from build123d import *

# Parameters (mm, degrees)
RESSALTO_EXTRUS_O1_DEPTH                             = 4
FILETE1_R                                            = 4
CHANFRO1_SIZE                                        = 1
FURO_DE_DI_METRO_6_0_6_1_D                           = 6
ESCAREADO_PARA_PARAFUSO_COM_CABE_A_ESCAR_D           = 3.4
ESCAREADO_PARA_PARAFUSO_COM_CABE_A_ESCAR_CSINK_D     = 6.3
ESCAREADO_PARA_PARAFUSO_COM_CABE_A_ESCAR_CSINK_ANGLE = 90
BROCA_DE_ROSQUEAR_PARA_TARRAXA_DE_M21_D              = 1.6
BROCA_DE_ROSQUEAR_PARA_TARRAXA_DE_M21_DEPTH          = 10
BROCA_DE_ROSQUEAR_PARA_TARRAXA_DE_M21_TIP            = 0.480688495
ESCAREADO_PARA_PARAFUSO_COM_CABE_A_E_2_D             = 3.4
ESCAREADO_PARA_PARAFUSO_COM_CABE_A_E_2_DEPTH         = 4
ESCAREADO_PARA_PARAFUSO_COM_CABE_A_E_2_CSINK_D       = 6.3
ESCAREADO_PARA_PARAFUSO_COM_CABE_A_E_2_CSINK_ANGLE   = 90
ESCAREADO_PARA_PARAFUSO_COM_CABE_A_E_2_TIP           = 1.021463052
ESBO_O10_R                                           = 4.55
CORTE_EXTRUS_O1_DEPTH                                = 3
FURO_DE_DI_METRO_3_5_3_5_1_D                         = 3.5


with BuildPart() as part:
    # Esboço1 → Ressalto-extrusão1 (new body)
    with BuildSketch(Plane.XY):
        Polygon((0, 0), (22, 0), (22, 60), (0, 50), align=None)
    extrude(amount=RESSALTO_EXTRUS_O1_DEPTH)

    # Filete1
    filete1_edges = [part.edges().sort_by_distance(p)[0] for p in [
        (0, 50, 2),
        (22, 60, 2),
    ]]
    fillet(filete1_edges, radius=FILETE1_R)

    # Chanfro1
    chanfro1_edges = [part.edges().sort_by_distance(p)[0] for p in [
        (22, 26.893991641, 4),
        (0, 23.712173459, 4),
        (9.344788223, 54.24763101, 4),
        (20.165542991, 57.151080598, 4),
        (0.636902684, 49.58988991, 4),
    ]]
    chamfer(chanfro1_edges, length=CHANFRO1_SIZE)

    # Furo de diâmetro Ø6.0 (6)1 (through all)
    with Locations(Plane(origin=(7.780869527, 38.393713373, 4), x_dir=(1, 0, 0), z_dir=(0, 0, 1))):
        with Locations((0, 0)):
            Hole(FURO_DE_DI_METRO_6_0_6_1_D / 2)

    # Escareado para parafuso com cabe_a escar (through all)
    with Locations(Plane(origin=(18, 7, 4), x_dir=(1, 0, 0), z_dir=(0, 0, 1))):
        with Locations((0, 0), (0, 7)):
            CounterSinkHole(ESCAREADO_PARA_PARAFUSO_COM_CABE_A_ESCAR_D / 2, ESCAREADO_PARA_PARAFUSO_COM_CABE_A_ESCAR_CSINK_D / 2, counter_sink_angle=ESCAREADO_PARA_PARAFUSO_COM_CABE_A_ESCAR_CSINK_ANGLE)

    # Broca de rosquear para tarraxa de M21
    with Locations(Plane(origin=(4, 0, 2), x_dir=(0, 0, -1), z_dir=(0, -1, 0))):
        with Locations((0, 0), (0, 8)):
            Hole(BROCA_DE_ROSQUEAR_PARA_TARRAXA_DE_M21_D / 2, depth=BROCA_DE_ROSQUEAR_PARA_TARRAXA_DE_M21_DEPTH)
            with Locations((0, 0, -(BROCA_DE_ROSQUEAR_PARA_TARRAXA_DE_M21_DEPTH + BROCA_DE_ROSQUEAR_PARA_TARRAXA_DE_M21_TIP / 2))):  # 118° drill point
                Cone(0, BROCA_DE_ROSQUEAR_PARA_TARRAXA_DE_M21_D / 2, BROCA_DE_ROSQUEAR_PARA_TARRAXA_DE_M21_TIP, mode=Mode.SUBTRACT)

    # Escareado para parafuso com cabe_a e 2
    with Locations(Plane(origin=(18, 30, 4), x_dir=(1, 0, 0), z_dir=(0, 0, 1))):
        with Locations((0, 0)):
            CounterSinkHole(ESCAREADO_PARA_PARAFUSO_COM_CABE_A_E_2_D / 2, ESCAREADO_PARA_PARAFUSO_COM_CABE_A_E_2_CSINK_D / 2, depth=ESCAREADO_PARA_PARAFUSO_COM_CABE_A_E_2_DEPTH, counter_sink_angle=ESCAREADO_PARA_PARAFUSO_COM_CABE_A_E_2_CSINK_ANGLE)
            with Locations((0, 0, -(ESCAREADO_PARA_PARAFUSO_COM_CABE_A_E_2_DEPTH + ESCAREADO_PARA_PARAFUSO_COM_CABE_A_E_2_TIP / 2))):  # 118° drill point
                Cone(0, ESCAREADO_PARA_PARAFUSO_COM_CABE_A_E_2_D / 2, ESCAREADO_PARA_PARAFUSO_COM_CABE_A_E_2_TIP, mode=Mode.SUBTRACT)

    # Esboço10 → Corte-extrusão1 (cut)
    with BuildSketch(Plane(origin=(0, 0, 0), x_dir=(-1, 0, 0), z_dir=(0, 0, -1))):
        with Locations((-7.780869527, 38.393713373)):
            Circle(ESBO_O10_R)
    extrude(amount=-CORTE_EXTRUS_O1_DEPTH, mode=Mode.SUBTRACT)

    # Furo de diâmetro Ø3.5 (3.5)1 (through all)
    with Locations(Plane(origin=(3, 14, 4), x_dir=(1, 0, 0), z_dir=(0, 0, 1))):
        with Locations((0, 0)):
            Hole(FURO_DE_DI_METRO_3_5_3_5_1_D / 2)


solid = part.part
Source: CAD feature listing. Evaluate the final solid. Frame: model axes, mm. A direction names the side the tool comes from. Give positions to 0.01 mm unless a question says otherwise; leave off trailing zeros. Write each loop counter-clockwise with the first axis right and the second up, starting at its lowest first coordinate (ties: lowest second). Pieces come first, ordered by that corner, then holes. Notation, with made-up numbers: (18, 59.5) - (67, 59.5) arc R13 cw to (67, 77.5) - close; hole circle Ø2 at (2.5, -4.5). An arc over 180 degrees is marked (long way). Write item = value, one per line. Start each with the question number.
Q1. Material intervals for probe 1 along Y at (x, z) = (18, 1); probe 2 along X at (y, z) = (3.25, 2); probe 3 along X at (y, z) = (7, 0.75), sorted ascending.
Q2. Cut plane B-B, the plane y = 36.5. Return loops of the section in (x, z), then the cut area to 3 significant figures.
Q3. Draft query along Z for faces 4 (the conical face through (3.88, 10.4, 1.94)), 5 (the cylindrical face through (0.654, 49.617, 1.521)), 6 (the conical face through (1.171, 49.278, 3.618)). Return one class per face: +Z half, -Z half, draft (parallel to the pull), parting line (faces both ways), or undercut.
Q4. Cut plane A-A, the plane y = 7. Return loops of the section in (x, z) (3 decimals), then the cut area to 3 significant figures.
Q5. Cut plane C-C, the plane x = 8.25. Return loops of the section in (y, z).
Q6. Cut plane D-D, the plane y = 30. Return loops of the section in (x, z) (3 decimals), then the cut area to 3 significant figures.
Q7. Pin query (flat end, axial travel): pin 1 Ø4 at (x, y) = (18, 7) entering from +Z. Return the tip coordinate at first contact, or that it passes through.
Q8. Reachability of faces 1 (the cylindrical face through (8.4, 42.9, 1.5)), 2 (the cylindrical face through (3.29, 5.07, 2.37)), 3 (the flat face through (0, 24, 1)) from +Z, -Z, +X, -X, +Y, -Y: full face, straight path, thin tool, end or side. Return the list, or none.
Computed values:
q1.probe_1 = 0 to 5.3, 8.7 to 12.3, 15.7 to 28.3, 31.7 to 57.79
q1.probe_2 = 0 to 3.2, 4.8 to 11.2, 12.8 to 22
q1.probe_3 = 0 to 16.3, 19.7 to 22
q2.outline = (0, 0) - (3.64, 0) - (3.64, 3) - (5.45, 3) - (5.45, 4) - (1, 4) - (0, 3) - close; (10.11, 3) - (11.92, 3) - (11.92, 0) - (22, 0) - (22, 3) - (21, 4) - (10.11, 4) - close
q2.area = 57.5 mm²
q3.face_4 = undercut
q3.face_5 = draft
q3.face_6 = +Z half
q4.outline = (0, 0) - (16.3, 0) - (16.3, 2.55) - (14.85, 4) - (1, 4) - (0, 3) - close; (19.7, 0) - (22, 0) - (22, 3) - (21.075, 3.925) - (19.7, 2.55) - close; hole circle Ø1.6 at (4, 2); hole circle Ø1.6 at (12, 2)
q4.area = 67.3 mm²
q5.outline = (0, 0) - (33.87, 0) - (33.87, 3) - (35.43, 3) - (35.43, 4) - (0, 4) - close; (41.36, 3) - (42.92, 3) - (42.92, 0) - (53.75, 0) - (53.75, 3) - (52.65, 4) - (41.36, 4) - close
q6.outline = (0, 0) - (16.3, 0) - (16.3, 2.55) - (14.85, 4) - (1, 4) - (0, 3) - close; (19.7, 0) - (22, 0) - (22, 3) - (21.075, 3.925) - (19.7, 2.55) - close
q6.area = 71.3 mm²
q7.pin_1 = 2.85
q8.face_1 = -Z
q8.face_2 = -Y
q8.face_3 = +Z, -Z, -X, +Y, -Y
